```python
from build123d import *

# Parameters (mm, degrees)
EXTRUDE_1_DEPTH     = 4
SKETCH_2_R          = 0.9
CUT_EXTRUDE_1_DEPTH = 52
SKETCH_3_W          = 2.000000328
SKETCH_3_H          = 4.999999888
EXTRUDE_2_DEPTH     = 1.5


with BuildPart() as part:
    # 草图1 → 凸台-拉伸1 (new body)
    with BuildSketch(Plane.XY):
        with BuildLine():
            Line((66.000003368, -0.999999465), (66.000003368, 1.000000862))
            ThreePointArc((66.000003368, 1.000000862), (65.646447605, 1.853552596), (66.500000656, 1.500000013))
            Line((66.500000656, 1.500000013), (69.000001997, 1.500000013))
            Line((69.000001997, 1.500000013), (69.000001997, 4.999999655))
            Line((69.000001997, 4.999999655), (40.0000019, 19.749999745))
            Line((40.0000019, 19.749999745), (37.000001874, 19.749999745))
            Line((37.000001874, 19.749999745), (37.000001874, 17.250002129))
            ThreePointArc((37.000001874, 17.250002129), (37.353555819, 16.396448761), (36.500001792, 16.750001116))
            Line((36.500001792, 16.750001116), (34.500001871, 16.750001116))
            ThreePointArc((34.500001871, 16.750001116), (33.646447808, 16.396448765), (34.000001848, 17.250002129))
            Line((34.000001848, 17.250002129), (34.000001848, 19.749999745))
            Line((34.000001848, 19.749999745), (31.000001822, 19.749999745))
            Line((31.000001822, 19.749999745), (31.000001822, 16.750001116))
            Line((31.000001822, 16.750001116), (34.000001848, 13.000000967))
            Line((34.000001848, 13.000000967), (34.000001848, 2.500000177))
            Line((34.000001848, 2.500000177), (19.492642954, 2.500000177))
            Line((19.492642954, 2.500000177), (10.000001639, 13.915917603))
            Line((10.000001639, 13.915917603), (10.000001639, 19.749999745))
            Line((10.000001639, 19.749999745), (7.000001147, 19.749999745))
            Line((7.000001147, 19.749999745), (7.000001147, 17.250002129))
            ThreePointArc((7.000001147, 17.250002129), (7.353556004, 16.396449439), (6.500001997, 16.750001116))
            Line((6.500001997, 16.750001116), (3.500001505, 16.750001116))
            ThreePointArc((3.500001505, 16.750001116), (2.646447808, 16.396449749), (3.000002354, 17.250002129))
            Line((3.000002354, 17.250002129), (3.000002354, 19.749999745))
            Line((3.000002354, 19.749999745), (0, 19.749999745))
            Line((0, 19.749999745), (0, -19.749999745))
            Line((0, -19.749999745), (3.000002354, -19.749999745))
            Line((3.000002354, -19.749999745), (3.000002354, -17.249999742))
            ThreePointArc((3.000002354, -17.249999742), (2.646448465, -16.39644732), (3.500001505, -16.749999719))
            Line((3.500001505, -16.749999719), (6.500001997, -16.749999719))
            ThreePointArc((6.500001997, -16.749999719), (7.353555348, -16.396447009), (7.000001147, -17.249999742))
            Line((7.000001147, -17.249999742), (7.000001147, -19.749999745))
            Line((7.000001147, -19.749999745), (10.000001639, -19.749999745))
            Line((10.000001639, -19.749999745), (10.000001639, -13.915917138))
            Line((10.000001639, -13.915917138), (19.492642954, -2.499999711))
            Line((19.492642954, -2.499999711), (34.000001848, -2.499999711))
            Line((34.000001848, -2.499999711), (34.000001848, -12.999999803))
            Line((34.000001848, -12.999999803), (31.000001822, -16.749999719))
            Line((31.000001822, -16.749999719), (31.000001822, -19.749999745))
            Line((31.000001822, -19.749999745), (34.000001848, -19.749999745))
            Line((34.000001848, -19.749999745), (34.000001848, -17.249999742))
            ThreePointArc((34.000001848, -17.249999742), (33.646448464, -16.396446335), (34.500001871, -16.749999719))
            Line((34.500001871, -16.749999719), (36.500001792, -16.749999719))
            ThreePointArc((36.500001792, -16.749999719), (37.353555162, -16.396446331), (37.000001874, -17.249999742))
            Line((37.000001874, -17.249999742), (37.000001874, -19.749999745))
            Line((37.000001874, -19.749999745), (40.0000019, -19.749999745))
            Line((40.0000019, -19.749999745), (69.000001997, -5.000000121))
            Line((69.000001997, -5.000000121), (69.000001997, -1.499999547))
            Line((69.000001997, -1.499999547), (66.500000656, -1.499999547))
            ThreePointArc((66.500000656, -1.499999547), (65.646447327, -1.853550818), (66.000003368, -0.999999465))
        make_face()
        Polygon((37.000001874, 13.000000967), (37.000001874, 1.500000013), (46.000001952, 1.500000013), (46.000001952, 4.500000505), (40.0000019, 14.666666044), align=None, mode=Mode.SUBTRACT)
        Polygon((42.838321999, -14.940624125), (49.000001512, -4.500000039), (49.000001512, -1.499999547), (63.000001013, -1.499999547), (64.000001177, -4.17735544), align=None, mode=Mode.SUBTRACT)
        Polygon((46.000001952, -1.499999547), (37.000001874, -1.499999547), (37.000001874, -12.999999803), (40.0000019, -14.666666277), (46.000001952, -4.500000039), align=None, mode=Mode.SUBTRACT)
        Polygon((63.000001013, 1.500000013), (64.000001177, 4.177356837), (42.838321999, 14.940623892), (49.000001512, 4.500000505), (49.000001512, 1.500000013), align=None, mode=Mode.SUBTRACT)
        Polygon((3.000002354, -13.749999693), (7.000001147, -13.749999693), (18.065146907, -1.59e-07), (7.000001147, 13.750000624), (3.000002354, 13.750000624), align=None, mode=Mode.SUBTRACT)
    extrude(amount=EXTRUDE_1_DEPTH)

    # 草图2 → 切除-拉伸1 (cut)
    with BuildSketch(Plane.XZ.offset(16.749999719)):
        with Locations((5.000002354, 2)):
            Circle(SKETCH_2_R)
    extrude(amount=-CUT_EXTRUDE_1_DEPTH, mode=Mode.SUBTRACT)

    # 草图3 → 凸台-拉伸2 (add)
    with BuildSketch(Plane.XY.offset(4)):
        Polygon((3.000002354, 12.413031189), (3.000002354, 13.750000624), (0, 12.680980144), (0, 10.680979816), align=None)
        with Locations((23.000001907, 2.33e-07)):
            Rectangle(SKETCH_3_W, SKETCH_3_H)
        Polygon((3.000002354, -13.749999693), (3.000002354, -12.413030723), (0, -10.680979816), (0, -12.680979678), align=None)
    extrude(amount=EXTRUDE_2_DEPTH)


solid = part.part
```
Could you check a few things on this model? Use its own coordinates, in mm. A direction names the side the tool comes from. Round coordinates to 2 decimals unless told otherwise and drop trailing zeros. Loops run counter-clockwise (first coordinate to the right, second up) from the corner with the lowest first, then second, coordinate; pieces in that order, holes last. Notation, with made-up numbers: (18, -37.75) -> (74, -37.75) arc R33 cw to (74, -4.75) -> close; hole circle Ø3 at (5, 3.25). An arc over 180 degrees is marked (long way). One line per question, with ' | ' between items.
(1) If we section it at D-D on x = 12: List the corners of the cut face in (y, z) for me.
Model answer:
outline: (-11.51, 0) -> (-7.54, 0) -> (-7.54, 4) -> (-11.51, 4) -> close; (7.54, 0) -> (11.51, 0) -> (11.51, 4) -> (7.54, 4) -> close
(2) If I drill on probe 1 along Y at (x, z) = (45.5, 1); probe 2 along X at (y, z) = (7, 2.5); probe 3 along X at (y, z) = (7.5, 3.35) (1 decimal), over which ranges is the centre line in solid material (lowest first)?
Model answer:
probe 1: y = -16.95 to -13.59, -10.43 to -5.35, -1.5 to 1.5, 5.35 to 10.43, 13.59 to 16.95 | probe 2: x = 0 to 3, 12.43 to 15.75, 34 to 37, 44.52 to 47.52, 58.45 to 65.07 | probe 3: x = 0 to 3, 12 to 15.3, 34 to 37, 44.2 to 47.2, 57.5 to 64.1
(3) If we section it at A-A on z = 2: Count the separate pieces of the cut face and the enclosed holes in it, and give its area (3 significant figures).
Model answer:
separate pieces: 2 | enclosed holes: 4 | area: 869 mm^2
(4) If we section it at C-C on y = -8: List the corners of the cut face in (x, z) for me.
Model answer:
outline: (0, 0) -> (3, 0) -> (3, 4) -> (0, 4) -> close; (11.63, 0) -> (14.92, 0) -> (14.92, 4) -> (11.63, 4) -> close; (34, 0) -> (37, 0) -> (37, 4) -> (34, 4) -> close; (43.93, 0) -> (46.93, 0) -> (46.93, 4) -> (43.93, 4) -> close; (56.48, 0) -> (63.1, 0) -> (63.1, 4) -> (56.48, 4) -> close
(5) For pin 1 Ø1.3 at (y, z) = (-18, 2) entering from +X; pin 2 Ø3 at (x, z) = (50.5, 3) entering from -Y; pin 3 Ø0.9 at (x, z) = (4.5, 1) entering from +Y, each with a flat end and sliding along its axis, tell me the tip position at first contact or that it passes through.
Model answer:
pin 1: stops at x = 44.72 | pin 2: stops at y = -15.17 | pin 3: stops at y = 16.75
(6) For faces 1 (the face through (32.48, 14.9, 1.97)), 2 (the face through (14.81, 8.13, 1.97)), 3 (the face through (46, 0, 4)), 4 (the face through (35, -16.75, 2)), 5 (the face through (34, 2, 0)), which set-ups out of +Z, -Z, +X, -X, +Y, -Y let a thin tool reach every point of the face, with its end or its side?
Model answer:
face 1: +Z, -Z | face 2: +Z, -Z, +Y | face 3: +Z, +X, +Y, -Y | face 4: +Z, -Z, -Y | face 5: -Z, +X, -X, +Y, -Y
(7) Thinking about a two-plate mould opening in X: for faces 6 (the face through (1.52, -11.56, 4.74)), 7 (the face through (1, 12, 5.5)), 8 (the face through (56, -1.5, 2)), which applies, released by +X, released by -X, zero draft, split by the parting line, or undercut?
Model answer:
face 6: released by +X | face 7: zero draft | face 8: undercut
(8) If we section it at B-B on x = 52: List the corners of the cut face in (y, z) for me, and give its area (3 significant figures).
Model answer:
outline: (-13.65, 0) -> (-10.28, 0) -> (-10.28, 4) -> (-13.65, 4) -> close; (-1.5, 0) -> (1.5, 0) -> (1.5, 4) -> (-1.5, 4) -> close; (10.28, 0) -> (13.65, 0) -> (13.65, 4) -> (10.28, 4) -> close | area: 38.9 mm^2
